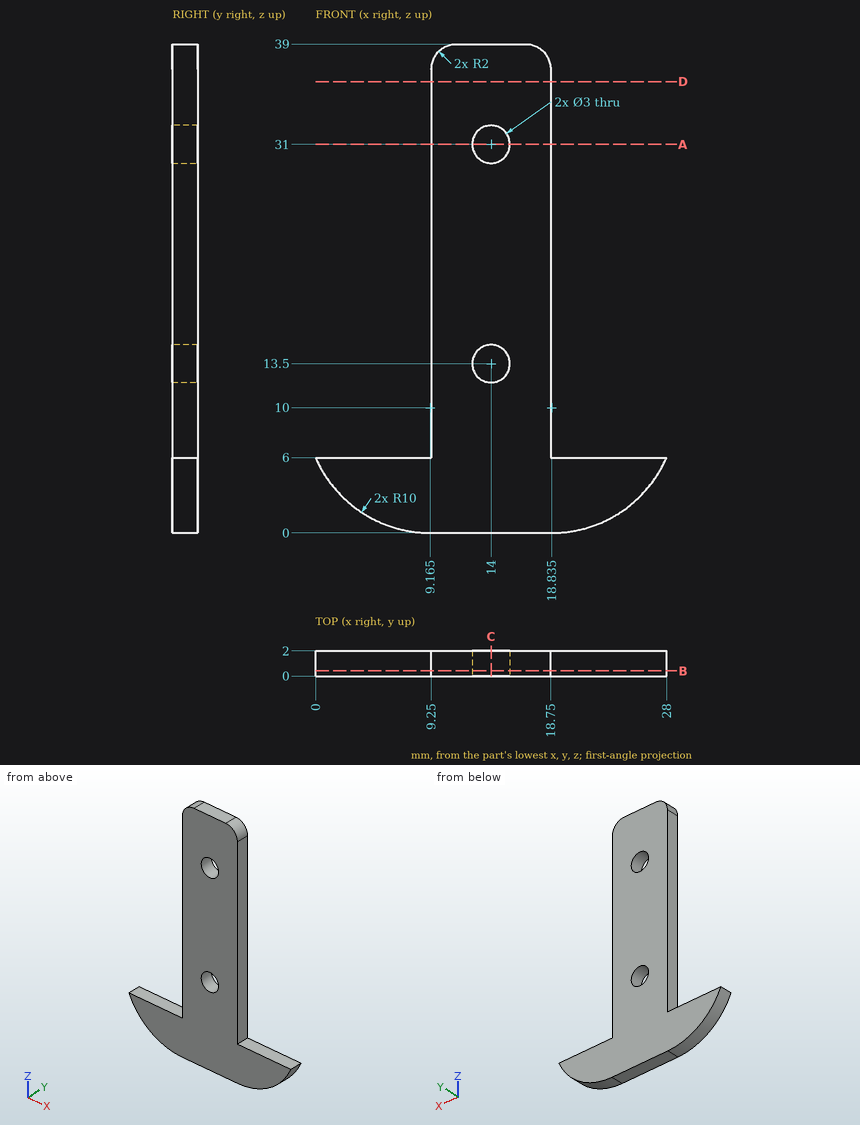
Geometry check sheet. Reference: drawing and pictorial views, mm from the part's lowest x, y, z. Round coordinates to 2 decimals unless told otherwise and drop trailing zeros. Order: outer loops, then holes, each group sorted by start corner. A loop starts at its lowest first (then second) coordinate and runs counter-clockwise, first axis right, second up.
Q1. Cross-section at D-D, the plane z = 36. Enter the section's corners in (x, y), plus the area to 3 significant figures.
Filled sheet:
outline: (9.25, 0) - (18.75, 0) - (18.75, 2) - (9.25, 2) - close
area: 19.0 mm2
Q2. Cross-section at B-B, the plane y = 0.4. Enter the section's corners in (x, z) (3 decimals), plus the area to 3 significant figures.
Filled sheet:
outline: (0, 6) arc R10 ccw to (9.165, 0) - (18.835, 0) arc R10 ccw to (28, 6) - (18.75, 6) - (18.75, 37) arc R2 ccw to (16.75, 39) - (11.25, 39) arc R2 ccw to (9.25, 37) - (9.25, 6) - close; hole circle Ø3 at (14, 13.5); hole circle Ø3 at (14, 31)
area: 435 mm2
Q3. Scan lines: L1, parallel to X at y = 1.65, z = 31; L2, parallel to Z at x = 14.75, y = 1.9; L3, parallel to X at y = 0.5, z = 15.5. Record each from-to range of solid material in increasing order.
Filled sheet:
L1: x = 9.25 to 12.5, 15.5 to 18.75
L2: z = 0 to 12.2, 14.8 to 29.7, 32.3 to 39
L3: x = 9.25 to 18.75
Q4. Cross-section at A-A, the plane z = 31. Enter the section's corners in (x, y), plus the area to 3 significant figures.
Filled sheet:
outline: (9.25, 0) - (12.5, 0) - (12.5, 2) - (9.25, 2) - close; (15.5, 0) - (18.75, 0) - (18.75, 2) - (15.5, 2) - close
area: 13.0 mm2
Q5. Depth check by flat-ended pin: P1, Ø1, axis at y = 1, z = 19.5, coming from the +X side; P2, Ø6, axis at x = 22.5, z = 12.5, coming from the +Y side; P3, Ø0.6, axis at x = 22, y = 0.5, coming from the +Z side. Enter the tip coordinate at first touch or a pass-through.
Filled sheet:
P1: stops at x = 18.75
P2: passes through
P3: stops at z = 6
Q6. Cross-section at C-C, the plane x = 14. Enter the section's corners in (y, z).
Filled sheet:
outline: (0, 0) - (2, 0) - (2, 12) - (0, 12) - close; (0, 15) - (2, 15) - (2, 29.5) - (0, 29.5) - close; (0, 32.5) - (2, 32.5) - (2, 39) - (0, 39) - close
